Can you work these out from the model? Positions are in its coordinate system, mm. A direction names the side the tool comes from. Coordinates: 2 decimals unless noted, no trailing zeros. Write each loop counter-clockwise with the first axis right and the second up, starting at its lowest first coordinate (ties: lowest second). Pieces come first, ordered by that corner, then holes.
```python
from build123d import *

# Parameters (mm, degrees)
CYLINDER003_W             = 5.25
CYLINDER003_H             = 4.13
CYLINDER003_ANGLE         = 90
CYLINDER002_R             = 1
CYLINDER002_DEPTH         = 13.55
FUSION002_PLACEMENT_ANGLE = 180
CYLINDER001_W             = 5.25
CYLINDER001_H             = 4.13
CYLINDER001_ANGLE         = 90
CYLINDER_R                = 1
CYLINDER_DEPTH            = 13.55
BOX_W                     = 47.1
BOX_H                     = 13.55
BOX_DEPTH                 = 43.1


with BuildPart() as obj1:
    # Cylinder003 → Cylinder003 (revolve)
    with BuildSketch(Plane(origin=(0, 4.13, 0), x_dir=(1, 0, 0), z_dir=(0, 0, -1))):
        with Locations((2.625, 2.065)):
            Rectangle(CYLINDER003_W, CYLINDER003_H)
    revolve(axis=Axis((0, 4.13, 0), (0, -1, 0)), revolution_arc=CYLINDER003_ANGLE)


with BuildPart() as obj2:
    # Cylinder002 → Cylinder002 (new body)
    with BuildSketch(Plane(origin=(2.5, 13.55, 2.5), x_dir=(1, 0, 0), z_dir=(0, -1, 0))):
        Circle(CYLINDER002_R)
    extrude(amount=CYLINDER002_DEPTH)

    # Fusion002: union obj1
    add(obj1.part)


with BuildPart() as obj2_1:
    # Fusion002 placement: moved
    add(obj2.part.moved(Location((47.1, 0, 43.1))).rotate(Axis((47.1, 0, 43.1), (0, 1, 0)), FUSION002_PLACEMENT_ANGLE))


with BuildPart() as obj3:
    # Cylinder001 → Cylinder001 (revolve)
    with BuildSketch(Plane(origin=(0, 4.13, 0), x_dir=(1, 0, 0), z_dir=(0, 0, -1))):
        with Locations((2.625, 2.065)):
            Rectangle(CYLINDER001_W, CYLINDER001_H)
    revolve(axis=Axis((0, 4.13, 0), (0, -1, 0)), revolution_arc=CYLINDER001_ANGLE)


with BuildPart() as fusion003:
    # Cylinder → Cylinder (new body)
    with BuildSketch(Plane(origin=(2.5, 13.55, 2.5), x_dir=(1, 0, 0), z_dir=(0, -1, 0))):
        Circle(CYLINDER_R)
    extrude(amount=CYLINDER_DEPTH)

    # Fusion001: union obj3
    add(obj3.part)

    # Fusion003: union obj2
    add(obj2_1.part)


with BuildPart() as ips7100v:
    # Box → Box (new body)
    with BuildSketch(Plane.XY):
        with Locations((23.55, 6.775)):
            Rectangle(BOX_W, BOX_H)
    extrude(amount=BOX_DEPTH)

    # Cut: cut Fusion003
    add(fusion003.part, mode=Mode.SUBTRACT)


with BuildPart() as ips7100v_1:
    # Cut placement: moved
    add(ips7100v.part.moved(Location((15, -33, 7.55))))


solid = ips7100v_1.part
```
1. If I drill on L1, parallel to X at y = -27, z = 10.05; L2, parallel to X at y = -20.25, z = 48; L3, parallel to Z at x = 59.6, y = -23.5, over which ranges is the centre line in solid material (lowest first)?
2. Which directions (+Z, -Z, +X, -X, +Y, -Y) give clear straight access to the entire face, cutting with the end or side of a thin tool? Please do faces 1 (the face through (61, -28.87, 49)), 2 (the face through (38, -33, 29)).
3. If we section it at B-B, the plane x = 17.5: List the corners of the cut face in (y, z) for me, plus the area to 3 significant figures.
4. We'd pull the mould along Z, two halves only. Please class faces 3 (the face through (18.753, -30.964, 11.221)), 4 (the face through (59.73, -24.09, 47.16)), 5 (the face through (18.424, -24.094, 9.667)), 6 (the face through (16, -28.87, 10)): released by +Z, released by -Z, zero draft, split by the parting line, or undercut.
5. If we section it at C-C, the plane y = -31.5: List the corners of the cut face in (x, z) for me.
6. I'm going to push flat-ended pins straight in: P1, Ø4, axis at x = 60, z = 49, coming from the -Y side; P2, Ø1.8, axis at x = 59.6, z = 48.15, coming from the -Y side. Where does each tip first touch, or does it pass through?
7. If we section it at A-A, the plane z = 10.05: List the corners of the cut face in (x, y) for me, plus the area to 3 significant figures.
Answers:
1. L1: x = 15 to 16.5, 18.5 to 62.1
1. L2: x = 15 to 58.61, 60.59 to 62.1
1. L3: z = 7.55 to 47.15, 49.15 to 50.65
2. face 1: +Z, +X, -Y
2. face 2: +Z, -Z, +X, -X, -Y
3. outline: (-33, 12.17) - (-28.87, 12.17) - (-28.87, 11.05) - (-19.45, 11.05) - (-19.45, 50.65) - (-33, 50.65) - close; (-28.87, 7.55) - (-19.45, 7.55) - (-19.45, 9.05) - (-28.87, 9.05) - close
3. area: 546 mm2
4. face 3: released by -Z
4. face 4: undercut
4. face 5: undercut
4. face 6: zero draft
5. outline: (15, 12.8) arc R5.25 cw to (20.25, 7.55) - (62.1, 7.55) - (62.1, 45.4) arc R5.25 cw to (56.85, 50.65) - (15, 50.65) - close
6. P1: stops at y = -28.87
6. P2: passes through
7. outline: (15, -28.87) - (16.5, -28.87) - (16.5, -19.45) - (15, -19.45) - close; (18.5, -28.87) - (19.62, -28.87) - (19.62, -33) - (62.1, -33) - (62.1, -19.45) - (18.5, -19.45) - close
7. area: 600 mm2
